from build123d import *

# Parameters (mm, degrees)
SKETCH2_W           = 18
SKETCH2_H           = 5
BOSS_EXTRUDE1_DEPTH = 5
CUT_EXTRUDE1_DEPTH  = 20.339079606
SKETCH4_W           = 18
SKETCH4_H           = 5
BOSS_EXTRUDE2_DEPTH = 2


with BuildPart() as part:
    # Sketch2 → Boss-Extrude1 (new body)
    with BuildSketch(Plane(origin=(0, 0, 0), x_dir=(1, 0, 0), z_dir=(0, 1, 0))):
        with Locations((9, 2.5)):
            Rectangle(SKETCH2_W, SKETCH2_H)
    extrude(amount=BOSS_EXTRUDE1_DEPTH)

    # Sketch3 → Cut-Extrude1 (cut, through all)
    with BuildSketch(Plane.XY):
        with BuildLine():
            Line((0, 5), (0, 0))
            Line((0, 0), (18, 0))
            Line((18, 0), (18, 2.3))
            ThreePointArc((18, 2.3), (8.806182909, 2.357886062), (0, 5))
        make_face()
    extrude(amount=-CUT_EXTRUDE1_DEPTH, mode=Mode.SUBTRACT)

    # Sketch4 → Boss-Extrude2 (add)
    with BuildSketch(Plane(origin=(0, 5, 0), x_dir=(1, 0, 0), z_dir=(0, 1, 0))):
        with Locations((9, 2.5)):
            Rectangle(SKETCH4_W, SKETCH4_H)
    extrude(amount=BOSS_EXTRUDE2_DEPTH)


solid = part.part
Work out the finished part from the listing and answer in its coordinate system (mm). Round coordinates to 2 decimals unless told otherwise and drop trailing zeros. Write each loop counter-clockwise with the first axis right and the second up, starting at its lowest first coordinate (ties: lowest second). Pieces come first, ordered by that corner, then holes. Notation, with made-up numbers: (70.5, 75.25) - (93.5, 75.25) arc R14 ccw to (93.5, 99.25) - close; hole circle Ø3 at (47, 83.5). An arc over 180 degrees is marked (long way). Answer in a Markdown table with one row per item. Add a question column.
1. Given pin 1 (2 mm diameter, centred on x = 8.5, z = -3, fed in from -Y), flat-ended and moving along its own axis, determine where the tip first touches the part or whether it passes through.
2. A cutting plane is placed at B-B, the plane y = 3.95. Determine the outline of the cut face in (x, z), and give its area (3 significant figures).
3. Find the intervals of material crossed by line 1 along Y through (x, z) = (13.5, -4.05); line 2 along Y through (x, z) = (3.5, -1.85); line 3 along X through (y, z) = (4.85, -1.8), in increasing order. Write a range as from..to.
4. A cutting plane is placed at A-A, the plane z = -2.25. Determine the outline of the cut face in (x, y).
Worked out:
| question | item | result |
|---|---|---|
| 1 | pin 1 | y = 2.26 |
| 2 | outline | (2.54, -5) - (18, -5) - (18, 0) - (2.54, 0) - close |
| 2 | area | 77.3 mm^2 |
| 3 | line 1 | 2..7 |
| 3 | line 2 | 3.62..7 |
| 3 | line 3 | 0.33..18 |
| 4 | outline | (0, 5) arc R32.35 ccw to (18, 2.3) - (18, 7) - (0, 7) - close |
